Part model, mm, in its own coordinate system. Coordinates: 2 decimals unless noted, no trailing zeros. Write each loop counter-clockwise with the first axis right and the second up, starting at its lowest first coordinate (ties: lowest second). Pieces come first, ordered by that corner, then holes. Notation, with made-up numbers: M 35,-34.75 L 53,-34.75 A30 ccw 53,-1.75 Z; hole C 71.5,53.5 d10. An arc over 180 degrees is marked long. Use a Markdown table: item, result. Add a question column.
Q1. Slice it at B-B on y = 399. Count the separate pieces of the cut face and the enclosed holes in it, then the cut area to 3 significant figures.
Q2. Wall check: L1, parallel to X at y = 404.5, z = 2.75; L2, parallel to X at y = 403.5, z = 12.75; L3, parallel to Y at x = 125, z = 13.5. Give the ranges that are in metal, low to high. Write a range as from..to.
Q3. Pin check, flat tips, straight feed: pin 1 Ø5 at (x, y) = (-255.5, 405) entering from -Z; pin 2 Ø13.5 at (x, y) = (-153.33, 403.33) entering from +Z. Stop position of each tip, or through.
Q4. Slice it at A-A on x = -125. Write the cut outline in (y, z), then the cut area to 3 significant figures.
Q5. Mould opens along X. For faces 1 (the flat face through (-390.5, 404, 9)), 2 (the cylindrical face through (-117.148, 400.078, 9.126)), 3 (the flat face through (390.5, 404, 9)), 4 (the flat face through (-5, 404, 18)) say: released by +X, released by -X, zero draft, split by the parting line, or undercut.
from build123d import *

# Parameters (mm, degrees)
SKETCH031_W          = 781
SKETCH031_H          = 27
PAD022_DEPTH         = 18
POCKET014_DEPTH      = 27.001
POCKET014_DEPTH_BACK = 0.001
SKETCH037_R          = 8.5
POCKET017_DEPTH      = 18.001
POCKET017_DEPTH_BACK = 0.001


with BuildPart() as part:
    # Sketch031 → Pad022 (new body)
    with BuildSketch(Plane.XY):
        Rectangle(SKETCH031_W, SKETCH031_H)
    extrude(amount=PAD022_DEPTH)

    # Sketch033 (on Face1 of Pad022) → Pocket014 (cut, two sides)
    with BuildSketch(Plane(origin=(0, 13.5, 0), x_dir=(-1, 0, 0), z_dir=(0, 1, 0))) as pocket014_sk:
        with BuildLine():
            ThreePointArc((-259.333333, 12), (-261.333333, 10), (-259.333333, 8))
            Line((-259.333333, 8), (-249.333333, 8))
            ThreePointArc((-249.333333, 8), (-247.333333, 10), (-249.333333, 12))
            Line((-249.333333, 12), (-259.333333, 12))
        make_face()
        with BuildLine():
            ThreePointArc((-29.333333, 12), (-31.333333, 10), (-29.333333, 8))
            Line((-29.333333, 8), (-19.333333, 8))
            ThreePointArc((-19.333333, 8), (-17.333333, 10), (-19.333333, 12))
            Line((-19.333333, 12), (-29.333333, 12))
        make_face()
        with BuildLine():
            ThreePointArc((19.333333, 12), (17.333333, 10), (19.333333, 8))
            Line((19.333333, 8), (29.333333, 8))
            ThreePointArc((29.333333, 8), (31.333333, 10), (29.333333, 12))
            Line((29.333333, 12), (19.333333, 12))
        make_face()
        with BuildLine():
            ThreePointArc((249.333333, 12), (247.333333, 10), (249.333333, 8))
            Line((249.333333, 8), (259.333333, 8))
            ThreePointArc((259.333333, 8), (261.333333, 10), (259.333333, 12))
            Line((259.333333, 12), (249.333333, 12))
        make_face()
    extrude(amount=-POCKET014_DEPTH, mode=Mode.SUBTRACT)
    extrude(pocket014_sk.sketch, amount=POCKET014_DEPTH_BACK, mode=Mode.SUBTRACT)

    # Sketch037 (on Face4 of Pocket014) → Pocket017 (cut, two sides)
    with BuildSketch(Plane.XY.offset(18)) as pocket017_sk:
        with Locations((-153.333333, -0.666667)):
            Circle(SKETCH037_R)
        with Locations((-125, -0.666667)):
            Circle(SKETCH037_R)
        with Locations((125, -0.666667)):
            Circle(SKETCH037_R)
        with Locations((153.333333, -0.666667)):
            Circle(SKETCH037_R)
    extrude(amount=-POCKET017_DEPTH, mode=Mode.SUBTRACT)
    extrude(pocket017_sk.sketch, amount=POCKET017_DEPTH_BACK, mode=Mode.SUBTRACT)


with BuildPart() as part_1:
    # Body022 placement: moved
    add(part.part.moved(Location((0, 404, 0))))


solid = part_1.part
Recorded:
| question | item | result |
|---|---|---|
| 1 | separate pieces | 5 |
| 1 | enclosed holes | 4 |
| 1 | area | 12,800 mm² |
| 2 | L1 | -390.5..-161.75, -144.91..-133.42, -116.58..116.58, 133.42..144.91, 161.75..390.5 |
| 2 | L2 | -390.5..-161.83, -144.83..-133.5, -116.5..116.5, 133.5..144.83, 161.83..390.5 |
| 2 | L3 | 390.5..394.83, 411.83..417.5 |
| 3 | pin 1 | z = 0 |
| 3 | pin 2 | through |
| 4 | outline | M 390.5,0 L 394.83,0 L 394.83,18 L 390.5,18 Z; M 411.83,0 L 417.5,0 L 417.5,18 L 411.83,18 Z |
| 4 | area | 180 mm² |
| 5 | face 1 | released by -X |
| 5 | face 2 | undercut |
| 5 | face 3 | released by +X |
| 5 | face 4 | zero draft |
